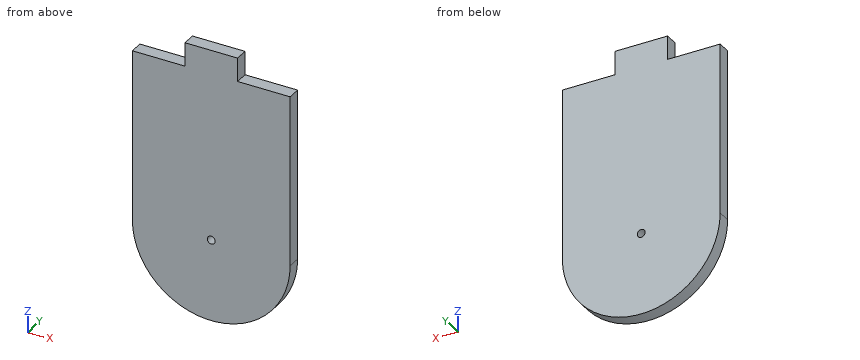
```python
from build123d import *

# Parameters (mm, degrees)
SKETCH1_W           = 60
SKETCH1_H           = 65
SKETCH1_W_2         = 20
SKETCH1_H_2         = 9
BOSS_EXTRUDE1_DEPTH = 5
SKETCH2_R           = 1.5
CUT_EXTRUDE1_DEPTH  = 6


with BuildPart() as part:
    # Sketch1 → Boss-Extrude1 (new body)
    with BuildSketch(Plane(origin=(0, 0, 0), x_dir=(1, 0, 0), z_dir=(0, 1, 0))):
        Rectangle(SKETCH1_W, SKETCH1_H)
        with Locations((0, -37)):
            Rectangle(SKETCH1_W_2, SKETCH1_H_2)
        with BuildLine():
            Line((-30, 32.5), (30, 32.5))
            ThreePointArc((30, 32.5), (0, 62.5), (-30, 32.5))
        make_face()
    extrude(amount=BOSS_EXTRUDE1_DEPTH)

    # Sketch2 → Cut-Extrude1 (cut, through all)
    with BuildSketch(Plane(origin=(0, 5, 0), x_dir=(1, 0, 0), z_dir=(0, 1, 0))):
        with Locations((0, 31.5)):
            Circle(SKETCH2_R)
    extrude(amount=-CUT_EXTRUDE1_DEPTH, mode=Mode.SUBTRACT)


solid = part.part
```
Geometry: final body of the model. Coordinates: model frame, mm. Round coordinates to 2 decimals unless told otherwise and drop trailing zeros. Order: outer loops, then holes, each group sorted by start corner. A loop starts at its lowest first (then second) coordinate and runs counter-clockwise, first axis right, second up. Notation, with made-up numbers: (79, 77.25) -> (133, 77.25) arc R15 ccw to (133, 95.25) -> close; hole circle Ø2 at (0.5, 41.25). An arc over 180 degrees is marked (long way). Use one line per item in the form item = value.
(1) Section B-B on x = 0. Return loops of the section in (y, z), and give its area (3 significant figures).
Results list:
outline = (0, -62.5) -> (5, -62.5) -> (5, -33) -> (0, -33) -> close; (0, -30) -> (5, -30) -> (5, 41.5) -> (0, 41.5) -> close
area = 505 mm^2
(2) Section C-C on y = 2.05. Return loops of the section in (x, z), and give its area (3 significant figures).
Results list:
outline = (-30, -32.5) arc R30 ccw to (30, -32.5) -> (30, 32.5) -> (10, 32.5) -> (10, 41.5) -> (-10, 41.5) -> (-10, 32.5) -> (-30, 32.5) -> close; hole circle Ø3 at (0, -31.5)
area = 5,490 mm^2
(3) Section D-D on x = 12.5. Return loops of the section in (y, z), and give its area (3 significant figures).
Results list:
outline = (0, -59.77) -> (5, -59.77) -> (5, 32.5) -> (0, 32.5) -> close
area = 461 mm^2
(4) Ray query, probe 1 along Z at (x, y) = (0, 3.45); probe 2 along X at (y, z) = (1.6, -31.5); probe 3 along Z at (x, y) = (-1, 0.25). Return the intervals inside material, ascending. Write a range as [from, to].
Results list:
probe_1 = [-62.5, -33], [-30, 41.5]
probe_2 = [-30, -1.5], [1.5, 30]
probe_3 = [-62.48, -32.62], [-30.38, 41.5]
(5) Section A-A on z = -31.5. Return loops of the section in (x, y), and give its area (3 significant figures).
Results list:
outline = (-30, 0) -> (-1.5, 0) -> (-1.5, 5) -> (-30, 5) -> close; (1.5, 0) -> (30, 0) -> (30, 5) -> (1.5, 5) -> close
area = 285 mm^2
(6) First-contact query: pin 1 Ø2.5 at (y, z) = (1.5, 35.5) entering from +X; pin 2 Ø1.5 at (x, y) = (-1.5, 2) entering from -Z; pin 3 Ø3 at (y, z) = (1, -49.5) entering from +X. Flat tips, straight axial feed; report the tip coordinate or a pass-through.
Results list:
pin_1 = 10
pin_2 = -62.49
pin_3 = 25.69
